Read the model definition and answer for the solid it produces. Units are mm, in the model's axes. Face numbers are marked on the shaded views. A direction names the side the tool comes from. Round coordinates to 2 decimals unless told otherwise and drop trailing zeros. Write each loop counter-clockwise with the first axis right and the second up, starting at its lowest first coordinate (ties: lowest second). Pieces come first, ordered by that corner, then holes. Notation, with made-up numbers: (43, -21.75) - (57, -21.75) arc R21 ccw to (57, -13.75) - close; hole circle Ø5 at (-39, 16). An arc over 180 degrees is marked (long way). One line per item, written item: value. Start each with the question number.
(1) A cutting plane is placed at A-A, the plane y = 3.75. Determine the outline of the cut face in (x, z), plus the area to 3 significant figures.
(2) A cutting plane is placed at C-C, the plane x = 0. Determine the outline of the cut face in (y, z), plus the area to 3 significant figures.
(3) Flat-ended cylindrical pins translate along their axes: pin 1 Ø1 at (x, y) = (5.5, 7) entering from +Z; pin 2 Ø1 at (y, z) = (11.5, -25.5) entering from -X; pin 3 Ø3 at (x, y) = (9, 15.5) entering from -Z. Find the tip coordinate at first contact, or state that the pin passes through.
(4) For the marked faces 1 and 2, determine the directions among +Z, -Z, +X, -X, +Y, -Y from which every point of the face is accessible in a straight line to the end or side of a thin tool.
(5) Find the intervals of material crossed by L1, parallel to X at y = 14.25, z = -21; L2, parallel to Y at x = 2, z = -4; L3, parallel to Z at x = -2, y = 7.25, in increasing order.
(6) A cutting plane is placed at B-B, the plane z = -9.5. Determine the outline of the cut face in (x, y).
(7) The mould has two halves that part along Z. Classify the marked faces 3, 4 and 5: +Z half, -Z half, draft (parallel to the pull), parting line (faces both ways), or undercut.
Autodesk Inventor part; units mm, degrees
ref_plane "YZ Plane" through (0, 0, 0) normal (1, 0, 0) x (0, 1, 0)
ref_plane "XZ Plane" through (0, 0, 0) normal (0, 1, 0) x (-1, 0, 0)
ref_plane "XY Plane" through (0, 0, 0) normal (0, 0, 1) x (1, 0, 0)
sketch "Sketch1" plane through (0, 0, 0) normal (0, 1, 0) x (-1, 0, 0)
  line L0 (0, 0) -> (0, -23.5) construction
  line L1 (-11.25, 0) -> (-11.25, -23.5)
  line L2 (11.25, -23.5) -> (11.25, 0)
  arc A0 (11.25, 0) -> (-11.25, 0) centre (0, 0) ccw
  arc A1 (-11.25, -23.5) -> (11.25, -23.5) centre (0, -23.5) ccw
  point P0 (0, -11.75)
  dimension "d0" = 23.5
  dimension "d1" = 22.5
extrude "Extrusion1" add sketch "Sketch1" along normal blind 1
sketch "Sketch2" plane through (0, 1, 0) normal (0, 1, 0) x (1, 0, 0)
  arc A0 (11.25, 23.5) -> (-11.25, 23.5) centre (0, 23.5) ccw
  line L0 (0, 0) -> (0, 23.5) construction
  line L1 (11.25, 0) -> (11.25, 23.5)
  line L2 (-11.25, 23.5) -> (-11.25, 0)
  arc A1 (-11.25, 0) -> (11.25, 0) centre (0, 0) ccw
  arc A2 (11.25, 23.5) -> (-11.25, 23.5) centre (0, 23.5) ccw
  line L3 (0, 0) -> (0, 23.5) construction
  line L4 (10, 0) -> (10, 23.5)
  line L5 (-10, 23.5) -> (-10, 0)
  arc A3 (-10, 0) -> (10, 0) centre (0, 0) ccw
  arc A4 (10, 23.5) -> (-10, 23.5) centre (0, 23.5) ccw
  point P0 (0, 11.75)
  point P1 (0, 11.75)
  dimension "d4" = 20
extrude "Extrusion2" add sketch "Sketch2" along normal blind 19
properties part number "Dopje"
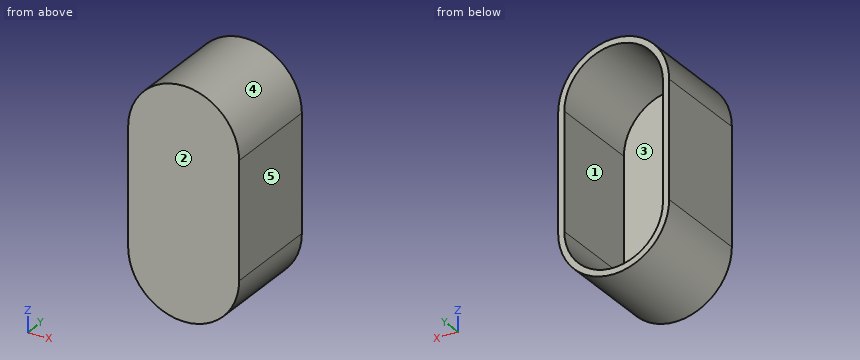
Here are the results:
1. outline: (-11.25, -23.5) arc R11.25 ccw to (11.25, -23.5) - (11.25, 0) arc R11.25 ccw to (-11.25, 0) - close; hole (-10, -23.5) arc R10 ccw to (10, -23.5) - (10, 0) arc R10 ccw to (-10, 0) - close
1. area: 142 mm²
2. outline: (0, -34.75) - (20, -34.75) - (20, -33.5) - (1, -33.5) - (1, 10) - (20, 10) - (20, 11.25) - (0, 11.25) - close
2. area: 93.5 mm²
3. pin 1: z = 10.08
3. pin 2: x = -11.15
3. pin 3: z = -31.89
4. face 1: +Y
4. face 2: +Z, -Z, +X, -X, -Y
5. L1: -11.25 to -10, 10 to 11.25
5. L2: 0 to 1
5. L3: -34.57 to -33.3, 9.8 to 11.07
6. outline: (-11.25, 0) - (11.25, 0) - (11.25, 20) - (10, 20) - (10, 1) - (-10, 1) - (-10, 20) - (-11.25, 20) - close
7. face 3: undercut
7. face 4: +Z half
7. face 5: draft
